Geometry: final body of the model. Coordinates: model frame, mm. A direction names the side the tool comes from. Give positions to 0.01 mm unless a question says otherwise; leave off trailing zeros. Write each loop counter-clockwise with the first axis right and the second up, starting at its lowest first coordinate (ties: lowest second). Pieces come first, ordered by that corner, then holes.
Q1. Cut plane B-B on z = 5.25. Return the cut outline in (x, y), plus the area to 3 significant figures.
Q2. Reachability of faces 5 (the face through (72.85, 156.29, 3.2)), 6 (the face through (77.7, 159.78, -5.27)), 7 (the face through (60.82, 137.277, -0.098)) from +Z, -Z, +X, -X, +Y, -Y: full face, straight path, thin tool, end or side. Return the list, or none.
Q3. Cut plane D-D on y = 152.5. Return the cut outline in (x, z), plus the area to 3 significant figures.
Q4. Cut plane A-A on x = 61.5. Return the cut outline in (y, z), plus the area to 3 significant figures.
Q5. Cut plane C-C on z = -1.25. Return the cut outline in (x, y).
Q6. Line query: L1, parallel to X at y = 132, z = -7; L2, parallel to Z at x = 61.5, y = 138.5; L3, parallel to X at y = 137, z = 1.5. Output: solid intervals per line, ascending.
Q7. Draft query along X for faces 1 (the face through (72.45, 162.23, -5.27)), 2 (the face through (78.21, 166.95, 6.7)), 3 (the face through (75, 162, 3.5)), 4 (the face through (66.07, 134.83, -0.1)). Return one class per face: pulls with the +X half, pulls with the -X half, needs draft (parallel to the pull), parting line crosses it, or undercut.
Q8. Pin query (flat end, axial travel): pin 1 (3 mm diameter, centred on x = 76.87, y = 164.84, fed in from +Z); pin 2 (6 mm diameter, centred on x = 69.5, z = 1.5, fed in from -Y); pin 3 (12 mm diameter, centred on y = 138, z = -5.5, fed in from +X); pin 4 (6 mm diameter, centred on x = 64.5, z = -3.5, fed in from +Y). Return the tip coordinate at first contact, or that it passes through.
```python
from build123d import *

# Parameters (mm, degrees)
SKETCH1_R               = 60
BOSS_EXTRUDE1_DEPTH     = 100
CUT_EXTRUDE1_DEPTH      = 452.895569028
CUT_EXTRUDE1_DEPTH_BACK = 452.895569028
SKETCH2_R               = 30
SKETCH2_R_2             = 25
SKETCH9_R               = 60
CUT_EXTRUDE4_DEPTH      = 35
CUT_EXTRUDE5_DEPTH      = 457.59902747
SKETCH12_W              = 140
SKETCH12_H              = 275.29462827
CUT_EXTRUDE6_DEPTH      = 27.5
SCALE1_SCALE            = 0.1


with BuildPart() as part:
    # Sketch1 → Boss-Extrude1 (new, symmetric)
    with BuildSketch(Plane.XY):
        with BuildLine():
            ThreePointArc((172.761636695, 269.924958208), (126.785478522, 271.892336111), (95.725474797, 305.847510456))
            Line((95.725474797, 305.847510456), (-20.619062469, 56.345845126))
            ThreePointArc((-20.619062469, 56.345845126), (25.357095704, 54.378467222), (56.417099429, 20.423292878))
            Line((56.417099429, 20.423292878), (172.761636695, 269.924958208))
        make_face()
        with Locations((152.142574227, 326.270803333)):
            Circle(SKETCH1_R)
        Circle(SKETCH1_R)
    extrude(amount=BOSS_EXTRUDE1_DEPTH, both=True)

    # Sketch2 → Cut-Extrude1 (cut, two sides: drawn at the far end of the back side and taken through both)
    with BuildSketch(Plane.XY.offset(-CUT_EXTRUDE1_DEPTH_BACK)):
        Circle(SKETCH2_R)
        with Locations((152.142574227, 326.270803333)):
            Circle(SKETCH2_R_2)
    extrude(amount=CUT_EXTRUDE1_DEPTH + CUT_EXTRUDE1_DEPTH_BACK, mode=Mode.SUBTRACT)

    # Sketch9 → Cut-Extrude4 (cut, symmetric)
    with BuildSketch(Plane.XY):
        with Locations((152.142574227, 326.270803333)):
            Circle(SKETCH9_R)
    extrude(amount=CUT_EXTRUDE4_DEPTH, both=True, mode=Mode.SUBTRACT)

    # Sketch10 → Cut-Extrude5 (cut, through all)
    with BuildSketch(Plane(origin=(-38.518080949, 17.961276124, 0), x_dir=(0, 0, 1), z_dir=(-0.906307787036651, 0.42261826174069733, 0))):
        with BuildLine():
            Line((-35, 317.647314135), (-35, 272.647314135))
            ThreePointArc((-35, 272.647314135), (-32.071067812, 265.576246323), (-25, 262.647314135))
            Line((-25, 262.647314135), (0, 262.647314135))
            Line((0, 262.647314135), (25, 262.647314135))
            ThreePointArc((25, 262.647314135), (32.071067812, 265.576246323), (35, 272.647314135))
            Line((35, 272.647314135), (35, 317.647314135))
            Line((35, 317.647314135), (-35, 317.647314135))
        make_face()
    extrude(amount=-CUT_EXTRUDE5_DEPTH, mode=Mode.SUBTRACT)

    # Sketch12 → Cut-Extrude6 (cut)
    with BuildSketch(Plane(origin=(-38.518080949, 17.961276124, 0), x_dir=(0, 0, 1), z_dir=(-0.906307787036651, 0.42261826174069733, 0))):
        with Locations((0, 180)):
            Rectangle(SKETCH12_W, SKETCH12_H)
    cut_extrude6 = extrude(amount=-CUT_EXTRUDE6_DEPTH, mode=Mode.SUBTRACT)

    # Mirror1: Cut-Extrude6 across plane
    add(cut_extrude6.mirror(Plane(origin=(0, 0, 0), x_dir=(0, 0, 1), z_dir=(-0.906307787036651, 0.42261826174069733, 0))), mode=Mode.SUBTRACT)


with BuildPart() as part_1:
    # Scale1: scaled about (68.503201219, 146.905589092, 0)
    add(part.part.scale(SCALE1_SCALE).moved(Location((61.652881097, 132.215030183, 0))))


solid = part_1.part
```
Data:
1. outline: (59.59, 137.85) arc R6 ccw (long way) to (67.29, 134.26) - (64.8, 135.42) - (76.44, 160.37) - (78.93, 159.21) arc R6 ccw (long way) to (71.23, 162.8) - (73.72, 161.64) - (62.08, 136.69) - close; hole circle Ø6 at (61.65, 132.22); hole circle Ø5 at (76.87, 164.84)
1. area: 240 mm2
2. face 5: +X, +Y
2. face 6: -Y
2. face 7: +Y
3. outline: (66.42, -10) - (75.8, -10) - (75.8, -7) - (72.77, -7) - (72.77, 7) - (75.8, 7) - (75.8, 10) - (66.42, 10) - (66.42, 7) - (69.46, 7) - (69.46, -7) - (66.42, -7) - close
3. area: 103 mm2
4. outline: (126.22, -10) - (129.22, -10) - (129.22, 10) - (126.22, 10) - close; (135.21, -10) - (141.94, -10) - (141.94, -7) - (136.96, -7) - (136.96, 7) - (141.94, 7) - (141.94, 10) - (135.21, 10) - close
4. area: 125 mm2
5. outline: (59.59, 137.85) arc R6 ccw (long way) to (67.29, 134.26) - (64.8, 135.42) - (74.11, 155.39) - (71.39, 156.65) - (62.08, 136.69) - close; hole circle Ø6 at (61.65, 132.22)
6. L1: x = 55.66 to 58.66, 64.65 to 67.65
6. L2: z = -10 to -7, 7 to 10
6. L3: x = 58.03 to 61.41, 62.23 to 65.54
7. face 1: pulls with the -X half
7. face 2: undercut
7. face 3: needs draft
7. face 4: pulls with the +X half
8. pin 1: passes through
8. pin 2: stops at y = 128.68
8. pin 3: stops at x = 71.75
8. pin 4: stops at y = 148.3
